```python
from build123d import *

# Parameters (mm, degrees)
BASPROSKE_W        = 3
BASPROSKE_H        = 12.75
TOOTHCUT_DEPTH     = 19.27908641
TEETHCUTS_COUNT    = 15
TEETHCUTS_ANGLE    = 336
BORSKE_R           = 2
BORE_DEPTH         = 50.0000508
BOSS_EXTRU_1_START = -3
BOSS_EXTRU_1_DEPTH = 3


with BuildPart() as part:
    # BasProSke → Base-Revolve (revolve)
    with BuildSketch(Plane(origin=(0, 0, 0), x_dir=(1, 0, 0), z_dir=(0, 1, 0)), mode=Mode.PRIVATE) as base_revolve_sk:
        with Locations((1.5, 6.375)):
            Rectangle(BASPROSKE_W, BASPROSKE_H)
    revolve(base_revolve_sk.sketch.rotate(Axis((-10, 0, 0), (1, 0, 0)), 180), axis=Axis((-10, 0, 0), (1, 0, 0)))

    # TooCutSke → ToothCut (cut, through all)
    with BuildSketch(Plane(origin=(0, 0, 0), x_dir=(0, 0, -1), z_dir=(1, 0, 0))):
        with BuildLine():
            ThreePointArc((0.791546546, 9.340520867), (0, 9.374), (-0.791546546, 9.340520867))
            ThreePointArc((-0.791546546, 9.340520867), (-1.235070734, 11.110218102), (-2.344732916, 12.558386549))
            ThreePointArc((-2.344732916, 12.558386549), (0, 12.7754), (2.344732916, 12.558386549))
            ThreePointArc((2.344732916, 12.558386549), (1.235070734, 11.110218102), (0.791546546, 9.340520867))
        make_face()
    toothcut = extrude(amount=TOOTHCUT_DEPTH, mode=Mode.SUBTRACT)

    # TeethCuts: ToothCut ×15 about axis
    teethcuts_axis = Axis((-10, 0, 0), (1, 0, 0))
    for i in range(1, TEETHCUTS_COUNT):
        add(toothcut.rotate(teethcuts_axis, i * TEETHCUTS_ANGLE / (TEETHCUTS_COUNT - 1)), mode=Mode.SUBTRACT)

    # BorSke → Bore (cut, symmetric)
    with BuildSketch(Plane(origin=(0, 0, 0), x_dir=(0, 0, -1), z_dir=(1, 0, 0))):
        with Locations(Location((0, 0, 0), (0, 0, 180))):
            Circle(BORSKE_R)
    extrude(amount=BORE_DEPTH, both=True, mode=Mode.SUBTRACT)

    # Esquisse1 → Boss.-Extru.1 (add)
    with BuildSketch(Plane.ZY.offset(BOSS_EXTRU_1_START)):
        with BuildLine():
            Line((1, 1.732050808), (1, -1.732050808))
            ThreePointArc((1, -1.732050808), (2, 0), (1, 1.732050808))
        make_face()
    extrude(amount=BOSS_EXTRU_1_DEPTH)


solid = part.part
```
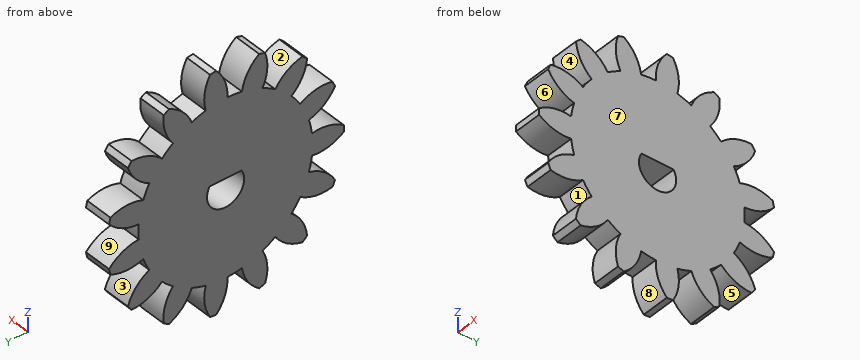
Read the model definition and answer for the solid it produces. Units are mm, in the model's axes. Face numbers are marked on the shaded views. A direction names the side the tool comes from. Give positions to 0.01 mm unless a question says otherwise; leave off trailing zeros. Write each loop counter-clockwise with the first axis right and the second up, starting at its lowest first coordinate (ties: lowest second). Pieces come first, ordered by that corner, then holes. Notation, with made-up numbers: (24, -39) -> (70, -39) arc R10 cw to (70, -21) -> close; hole circle Ø8 at (-37.75, 55.5). An arc over 180 degrees is marked (long way). Answer as a JSON object with one key per item and string values.
1) Straight lines are drawn through the part: probe 1 along Y at (x, z) = (2.25, 9.75); probe 2 along Y at (x, z) = (2.7, 11); probe 3 along Z at (x, y) = (2.8, -5.25). For each, find the intervals that lie inside material, in ascending order. Write a range as from..to.
Findings below:
{"probe 1": "y = -4.42..-1.88, -0.2..2.26, 4.24..6.66", "probe 2": "y = -4.48..-2.44, 0.01..2.25, 5.66..6.45", "probe 3": "z = -7.77..7.77"}
2) For a pull along Y with two mould halves and no side action, classify the marked faces 6, 7, 8 and 9 as pulls with the +Y half, pulls with the -Y half, needs draft (parallel to the pull), parting line crosses it, or undercut.
Findings below:
{"face 6": "pulls with the -Y half", "face 7": "needs draft", "face 8": "undercut", "face 9": "pulls with the +Y half"}
3) Section B-B on y = 9.75 is taken. Write down the section's boundary in (x, z).
Findings below:
{"outline": "(0, -7.75) -> (3, -7.75) -> (3, -5.77) -> (0, -5.77) -> close; (0, -3.33) -> (3, -3.33) -> (3, -0.83) -> (0, -0.83) -> close; (0, 0.83) -> (3, 0.83) -> (3, 3.33) -> (0, 3.33) -> close; (0, 5.77) -> (3, 5.77) -> (3, 7.75) -> (0, 7.75) -> close"}
4) A tool of negligible diameter and unlimited length cuts with its end or side. For the marked faces 1, 2, 3, 4 and 5, from which of +Z, -Z, +X, -X, +Y, -Y can it reach the whole face along a straight path? Write none if from no direction.
Findings below:
{"face 1": "+X, -X", "face 2": "+Z, +X, -X", "face 3": "+X, -X, +Y", "face 4": "+X, -X, -Y", "face 5": "-Z, +X, -X"}
5) Section A-A on z = 0 is taken. Write down the section's boundary in (x, y).
Findings below:
{"outline": "(0, -12.75) -> (3, -12.75) -> (3, -2) -> (0, -2) -> close; (0, 2) -> (3, 2) -> (3, 9.37) -> (0, 9.37) -> close"}
6) A flat-ended cylindrical pin translates along its axis: pin 1 Ø1 at (x, y) = (2, 4) entering from +Z. Find the tip coordinate at first contact, or state that the pin passes through.
Findings below:
{"pin 1": "stops at z = 10.07"}
7) Section C-C on z = -3.75 is taken. Write down the section's boundary in (x, y), then the cut area to 3 significant figures.
Findings below:
{"outline": "(0, -10.89) -> (3, -10.89) -> (3, 8.59) -> (0, 8.59) -> close", "area": "58.4 mm^2"}
